```python
from build123d import *

# Parameters (mm, degrees)
CROQUIS1_W              = 41
CROQUIS1_H              = 40
SALIENTE_EXTRUIR1_DEPTH = 20
CROQUIS2_R              = 3.5
SALIENTE_EXTRUIR2_DEPTH = 1.5
SALIENTE_EXTRUIR3_START = 1.5
CROQUIS3_R              = 3.5
SALIENTE_EXTRUIR3_DEPTH = 1.5
CROQUIS4_R              = 10.5
SALIENTE_EXTRUIR4_DEPTH = 4
SALIENTE_EXTRUIR5_START = 4
CROQUIS5_R              = 10.5
SALIENTE_EXTRUIR5_DEPTH = 4
SALIENTE_EXTRUIR8_START = 1.5
CROQUIS8_R              = 3.5
SALIENTE_EXTRUIR8_DEPTH = 1.5
CROQUIS9_R              = 3.5
SALIENTE_EXTRUIR9_DEPTH = 1.5


with BuildPart() as part:
    # Croquis1 → Saliente-Extruir1 (new body)
    with BuildSketch(Plane.XY):
        Rectangle(CROQUIS1_W, CROQUIS1_H)
    extrude(amount=SALIENTE_EXTRUIR1_DEPTH)

    # Croquis2 → Saliente-Extruir2 (add)
    with BuildSketch(Plane(origin=(20.5, 0, 0), x_dir=(0, 0, -1), z_dir=(1, 0, 0))):
        with Locations(Location((-10, -10, 0), (0, 0, 180))):
            Circle(CROQUIS2_R)
    extrude(amount=SALIENTE_EXTRUIR2_DEPTH)

    # Croquis3 → Saliente-Extruir3 (add)
    with BuildSketch(Plane.ZY.offset(20.5).offset(SALIENTE_EXTRUIR3_START)):
        with Locations((10, -10)):
            Circle(CROQUIS3_R)
    extrude(amount=-SALIENTE_EXTRUIR3_DEPTH)

    # Croquis4 → Saliente-Extruir4 (add)
    with BuildSketch(Plane(origin=(22, 0, 0), x_dir=(0, 0, -1), z_dir=(1, 0, 0))):
        with Locations((-10, -10)):
            Circle(CROQUIS4_R)
    extrude(amount=SALIENTE_EXTRUIR4_DEPTH)

    # Croquis5 → Saliente-Extruir5 (add)
    with BuildSketch(Plane.ZY.offset(22).offset(SALIENTE_EXTRUIR5_START)):
        with Locations(Location((10, -10, 0), (0, 0, 180))):
            Circle(CROQUIS5_R)
    extrude(amount=-SALIENTE_EXTRUIR5_DEPTH)

    # Croquis8 → Saliente-Extruir8 (add)
    with BuildSketch(Plane.ZY.offset(26).offset(SALIENTE_EXTRUIR8_START)):
        with Locations((10, -10)):
            Circle(CROQUIS8_R)
    extrude(amount=-SALIENTE_EXTRUIR8_DEPTH)

    # Croquis9 → Saliente-Extruir9 (add)
    with BuildSketch(Plane(origin=(26, 0, 0), x_dir=(0, 0, -1), z_dir=(1, 0, 0))):
        with Locations(Location((-10, -10, 0), (0, 0, 180))):
            Circle(CROQUIS9_R)
    extrude(amount=SALIENTE_EXTRUIR9_DEPTH)


solid = part.part
```
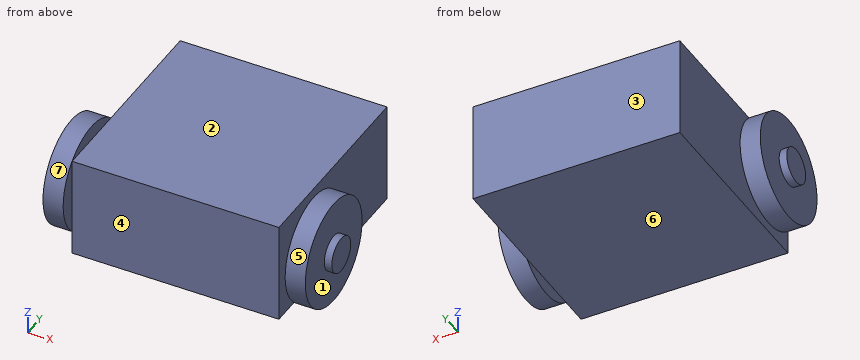
CAD build for the part. Positions are in the model's coordinates, mm. Face numbers are marked on the shaded views. A direction names the side the tool comes from. Coordinates: 2 decimals unless noted, no trailing zeros. Write each loop counter-clockwise with the first axis right and the second up, starting at its lowest first coordinate (ties: lowest second). Pieces come first, ordered by that corner, then holes.
(1) Cut at B-B, the plane z = 10. List the corners of the cut face in (x, y).
(2) 3-axis set-ups, long thin cutter, end or side, ignore diameter. For the marked faces 4, 5, 6 and 7: which of +Z, -Z, +X, -X, +Y, -Y reach the whole face in a straight line?
(3) Cut at A-A, the plane z = 2.5. List the corners of the cut face in (x, y), and give its area (3 significant figures).
(4) Cut at C-C, the plane x = -17.5. List the corners of the cut face in (y, z).
(5) Flat gauge pins, fed straight in: pin 1 (3 mm diameter, centred on y = -16, z = 7.5, fed in from +X); pin 2 (6.5 mm diameter, centred on y = -15, z = 13.5, fed in from -X); pin 3 (5 mm diameter, centred on y = 15.5, z = 3.5, fed in from +X); pin 4 (2 mm diameter, centred on x = -15, y = 8, fed in from -Z). Where does each tip first touch, or does it go through?
(6) Drill centre lines: probe 1 along X at (y, z) = (-7, 1); probe 2 along X at (y, z) = (6, 1.25); probe 3 along Y at (x, z) = (-12, 3.75). Where is each one in solid material? Low to high.
(7) Two-plate mould, pull along X, no slides. Class the marked faces 1, 2 and 3: +X half, -X half, draft (parallel to the pull), parting line (faces both ways), or undercut.
(8) Cut at D-D, the plane y = 10. List the corners of the cut face in (x, z).
Geometry says:
1. outline: (-27.5, -13.5) - (-26, -13.5) - (-26, -20.5) - (-22, -20.5) - (-22, -13.5) - (-20.5, -13.5) - (-20.5, -20) - (20.5, -20) - (20.5, -13.5) - (22, -13.5) - (22, -20.5) - (26, -20.5) - (26, -13.5) - (27.5, -13.5) - (27.5, -6.5) - (26, -6.5) - (26, 0.5) - (22, 0.5) - (22, -6.5) - (20.5, -6.5) - (20.5, 20) - (-20.5, 20) - (-20.5, -6.5) - (-22, -6.5) - (-22, 0.5) - (-26, 0.5) - (-26, -6.5) - (-27.5, -6.5) - close
2. face 4: +Z, -Z, -Y
2. face 5: +X
2. face 6: -Z, +Y, -Y
2. face 7: -X
3. outline: (-26, -17.35) - (-22, -17.35) - (-22, -2.65) - (-26, -2.65) - close; (-20.5, -20) - (20.5, -20) - (20.5, 20) - (-20.5, 20) - close; (22, -17.35) - (26, -17.35) - (26, -2.65) - (22, -2.65) - close
3. area: 1,760 mm2
4. outline: (-20, 0) - (20, 0) - (20, 20) - (-20, 20) - close
5. pin 1: stops at x = 26
5. pin 2: stops at x = -27.5
5. pin 3: stops at x = 20.5
5. pin 4: stops at z = 0
6. probe 1: x = -26 to -22, -20.5 to 20.5, 22 to 26
6. probe 2: x = -20.5 to 20.5
6. probe 3: y = -20 to 20
7. face 1: +X half
7. face 2: undercut
7. face 3: draft
8. outline: (-20.5, 0) - (20.5, 0) - (20.5, 20) - (-20.5, 20) - close
